Read the model definition and answer for the solid it produces. Units are mm, in the model's axes. A direction names the side the tool comes from. Coordinates: 2 decimals unless noted, no trailing zeros. Order: outer loops, then holes, each group sorted by start corner. A loop starts at its lowest first (then second) coordinate and runs counter-clockwise, first axis right, second up. Notation, with made-up numbers: (3, -28) - (38, -28) arc R28 ccw to (38, 5) - close; hole circle Ø11 at (18.25, 17.25). An arc over 180 degrees is marked (long way). Write item = value, one per line.
from build123d import *

# Parameters (mm, degrees)
BOSS_EXTRUDE1_DEPTH = 160
SKETCH2_R           = 4
SKETCH2_R_2         = 4.5
CUT_EXTRUDE2_DEPTH  = 5
SKETCH3_R           = 2.5
SKETCH3_R_2         = 4.5
CUT_EXTRUDE3_DEPTH  = 10


with BuildPart() as part:
    # Sketch1 → Boss-Extrude1 (new body)
    with BuildSketch(Plane(origin=(0, 0, 0), x_dir=(1, 0, 0), z_dir=(0, 1, 0))):
        Polygon((0, 20), (2.5, 20), (2.5, 25), (0, 25), (0, 38.5), (10, 38.5), (10, 0), (0, 0), (-4, 0), (-4, 15), (0, 15), align=None)
    extrude(amount=BOSS_EXTRUDE1_DEPTH)

    # Sketch2 → Cut-Extrude2 (cut)
    with BuildSketch(Plane(origin=(10, 0, 0), x_dir=(0, 0, -1), z_dir=(1, 0, 0))):
        with Locations((30.5, 145)):
            Circle(SKETCH2_R)
        with Locations((30.5, 85)):
            Circle(SKETCH2_R)
        with Locations((30.5, 25)):
            Circle(SKETCH2_R)
        with Locations((30.5, 12)):
            Circle(SKETCH2_R_2)
    extrude(amount=-CUT_EXTRUDE2_DEPTH, mode=Mode.SUBTRACT)

    # Sketch3 → Cut-Extrude3 (cut, through all)
    with BuildSketch(Plane(origin=(5, 0, 0), x_dir=(0, 0, -1), z_dir=(1, 0, 0))):
        with Locations((30.5, 145)):
            Circle(SKETCH3_R)
        with Locations((30.5, 85)):
            Circle(SKETCH3_R)
        with Locations((30.5, 25)):
            Circle(SKETCH3_R)
        with Locations((30.5, 12)):
            Circle(SKETCH3_R_2)
    extrude(amount=-CUT_EXTRUDE3_DEPTH, mode=Mode.SUBTRACT)


solid = part.part
1) Flat-ended cylindrical pins translate along their axes: pin 1 Ø10.5 at (y, z) = (25, -30.5) entering from -X; pin 2 Ø4 at (y, z) = (83.5, -30.5) entering from +X. Find the tip coordinate at first contact, or state that the pin passes through.
Returned:
pin_1 = 0
pin_2 = 5
2) The part is cut by section B-B (x = 7). Determine the outline of the cut face in (y, z).
Returned:
outline = (0, -38.5) - (160, -38.5) - (160, 0) - (0, 0) - close; hole circle Ø9 at (12, -30.5); hole circle Ø8 at (25, -30.5); hole circle Ø8 at (85, -30.5); hole circle Ø8 at (145, -30.5)
3) The part is cut by section D-D (y = 130.5). Determine the outline of the cut face in (x, z), and give its area (4 significant figures).
Returned:
outline = (-4, -15) - (0, -15) - (0, -20) - (2.5, -20) - (2.5, -25) - (0, -25) - (0, -38.5) - (10, -38.5) - (10, 0) - (-4, 0) - close
area = 432.5 mm^2
4) Straight lines are drawn through the part: line 1 along Y through (x, z) = (1.7, -30.5); line 2 along Y through (x, z) = (9.05, -30.5); line 3 along Z through (x, y) = (0.5, 72.5). For each, find the intervals that lie inside material, in ascending order. Write a range as from..to.
Returned:
line_1 = 0..7.5, 16.5..22.5, 27.5..82.5, 87.5..142.5, 147.5..160
line_2 = 0..7.5, 16.5..21, 29..81, 89..141, 149..160
line_3 = -38.5..-25, -20..0
5) The part is cut by section A-A (y = 12). Determine the outline of the cut face in (x, z), and give its area (4 significant figures).
Returned:
outline = (-4, -15) - (0, -15) - (0, -20) - (2.5, -20) - (2.5, -25) - (0, -25) - (0, -26) - (10, -26) - (10, 0) - (-4, 0) - close; (0, -38.5) - (10, -38.5) - (10, -35) - (0, -35) - close
area = 342.5 mm^2
6) The part is cut by section C-C (z = -30). Count the separate pieces of the cut face and the enclosed holes in it, and give its area (3 significant figures).
Returned:
separate_pieces = 5
enclosed_holes = 0
area = 1,320 mm^2
7) For faces 1 (the face through (-2, 79, -15)), 2 (the face through (1, 79, -20)), 3 (the face through (5, 22, -30)), determine the directions among +Z, -Z, +X, -X, +Y, -Y from which every point of the face is accessible in a straight line to the end or side of a thin tool.
Returned:
face_1 = -Z, -X, +Y, -Y
face_2 = -X, +Y, -Y
face_3 = +X
